Geometry check sheet. Reference: drawing and pictorial views, mm from the part's lowest x, y, z. Round coordinates to 2 decimals unless told otherwise and drop trailing zeros. Loops run counter-clockwise (first coordinate to the right, second up) from the corner with the lowest first, then second, coordinate; pieces in that order, holes last. Notation, with made-up numbers: (-3, 67) - (56, 67) arc R24 cw to (56, 86) - close; hole circle Ø3 at (-6.5, 9). An arc over 180 degrees is marked (long way). Put each result on its own line as item: value. Start each with the question number.
Item 1: Material ranges on line 1 along X through (y, z) = (5, 33.5); line 2 along Y through (x, z) = (0.3, 10) (1 decimal); line 3 along Y through (x, z) = (0.8, 28) (1 decimal), recorded low to high.
Item 2: Section check B-B, the plane y = 15.5. Record the cut outline in (x, z) (1 decimal).
Item 3: Draft check along Z on the marked faces 1, 2 and 3. Enter one of: pulls with the +Z half, pulls with the -Z half, needs draft (parallel to the pull), parting line crosses it, or undercut.
Item 4: Section check A-A, the plane z = 31. Record the cut outline in (x, y) (1 decimal).
Item 5: Section check C-C, the plane x = 1.95. Record the cut outline in (y, z) (1 decimal).
Item 6: Gauge pin test, flat ends, axial feed: pin 1 Ø2 at (x, z) = (2.5, 20.5) entering from +Y; pin 2 Ø4 at (y, z) = (21, 24.5) entering from -X; pin 3 Ø3 at (y, z) = (25.34, 43.26) entering from +X. Record the tip position at first contact, or that the pin passes through.
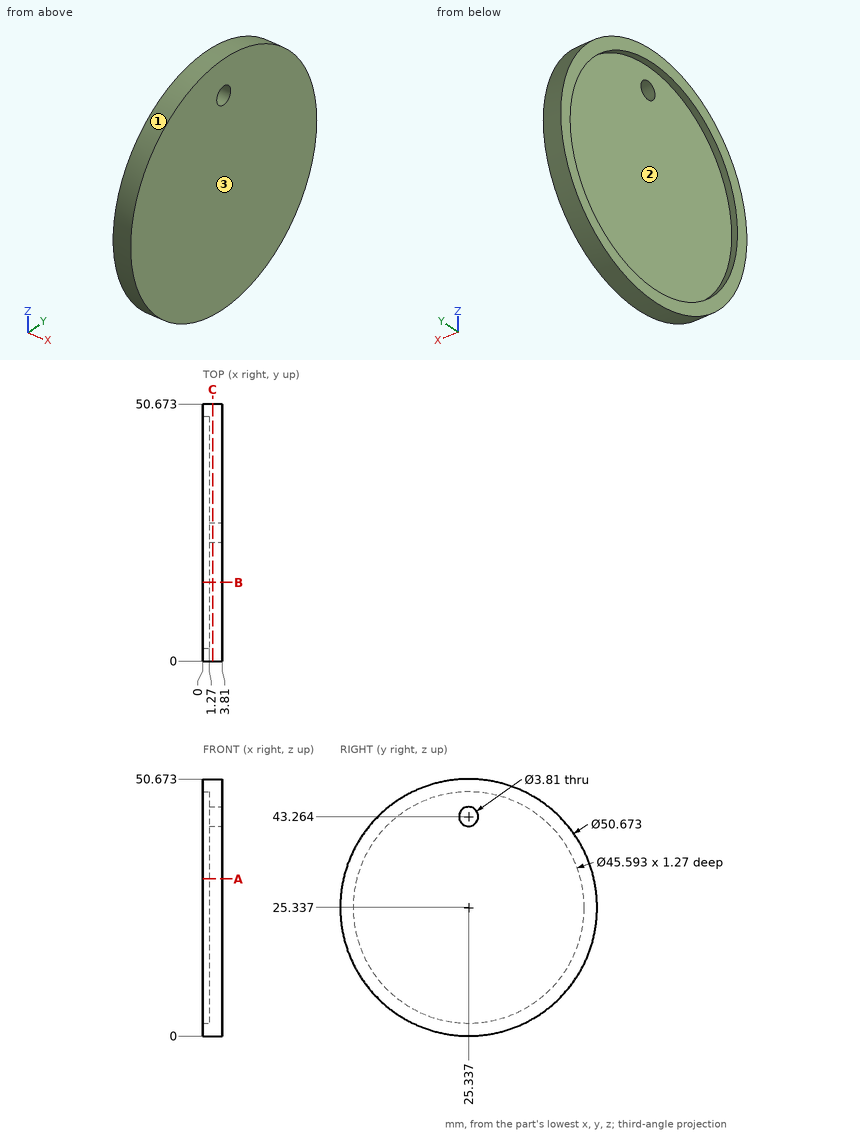
Check result:
1. line 1: 1.27 to 3.81
1. line 2: 5.2 to 8.5, 42.2 to 45.5
1. line 3: 0.1 to 2.7, 48 to 50.5
2. outline: (0, 2) - (3.8, 2) - (3.8, 48.7) - (0, 48.7) - (0, 45.9) - (1.3, 45.9) - (1.3, 4.8) - (0, 4.8) - close
3. face 1: parting line crosses it
3. face 2: undercut
3. face 3: needs draft
4. outline: (0, 0.6) - (3.8, 0.6) - (3.8, 50) - (0, 50) - (0, 47.4) - (1.3, 47.4) - (1.3, 3.3) - (0, 3.3) - close
5. outline: circle Ø50.7 at (25.3, 25.3); hole circle Ø3.8 at (25.3, 43.3)
6. pin 1: y = 50.38
6. pin 2: x = 1.27
6. pin 3: through
